from build123d import *

# Parameters (mm, degrees)
SKETCH1_W           = 15
SKETCH1_H           = 20
BOSS_EXTRUDE1_DEPTH = 20
FILLET1_R           = 7.5
CUT_EXTRUDE1_START  = -4.75
SKETCH3_R           = 8.5
CUT_EXTRUDE1_DEPTH  = 10.5
SKETCH4_R           = 2.5
CUT_EXTRUDE2_DEPTH  = 30.261749777
CUT_EXTRUDE3_DEPTH  = 3
SKETCH6_R           = 4
CUT_EXTRUDE4_DEPTH  = 3
CUT_EXTRUDE5_DEPTH  = 30.261749777
SKETCH8_R           = 8.5
CUT_EXTRUDE6_DEPTH  = 5
SKETCH9_R           = 2.5
CUT_EXTRUDE7_DEPTH  = 27.100766272
CUT_EXTRUDE8_START  = -1
CUT_EXTRUDE8_DEPTH  = 2.5
SKETCH11_R          = 1.5
CUT_EXTRUDE9_DEPTH  = 10
SKETCH12_W          = 15
SKETCH12_H          = 7
CUT_EXTRUDE10_DEPTH = 5
SKETCH13_W          = 15
SKETCH13_H          = 7
CUT_EXTRUDE11_DEPTH = 5
FILLET2_R           = 5


# Some blends are built 0.0001 mm under size
with BuildPart() as part:
    # Sketch1 → Boss-Extrude1 (new, symmetric)
    with BuildSketch(Plane.XY):
        Rectangle(SKETCH1_W, SKETCH1_H)
    extrude(amount=BOSS_EXTRUDE1_DEPTH, both=True)

    # Fillet1
    fillet1_edges = [part.edges().sort_by_distance(p)[0] for p in [
        (-7.5, 0, -20),
        (7.5, 0, -20),
    ]]
    fillet(fillet1_edges, radius=FILLET1_R - 0.0001)  # a hair under: the kernel refuses the full size

    # Sketch3 → Cut-Extrude1 (cut)
    with BuildSketch(Plane(origin=(0, 10, 0), x_dir=(1, 0, 0), z_dir=(0, 1, 0)).offset(CUT_EXTRUDE1_START)):
        with Locations((0, 12.5)):
            Circle(SKETCH3_R)
    extrude(amount=-CUT_EXTRUDE1_DEPTH, mode=Mode.SUBTRACT)

    # Sketch4 → Cut-Extrude2 (cut, through all)
    with BuildSketch(Plane(origin=(0, 10, 0), x_dir=(1, 0, 0), z_dir=(0, 1, 0))):
        with Locations(Location((0, 12.5, 0), (0, 0, 270))):
            Circle(SKETCH4_R)
    extrude(amount=-CUT_EXTRUDE2_DEPTH, mode=Mode.SUBTRACT)

    # Sketch5 → Cut-Extrude3 (cut)
    with BuildSketch(Plane(origin=(0, -10, 0), x_dir=(-1, 0, 0), z_dir=(0, -1, 0))):
        Polygon((-2.020725942, 16), (-4.041451884, 12.5), (-2.020725942, 9), (2.020725942, 9), (4.041451884, 12.5), (2.020725942, 16), align=None)
    extrude(amount=-CUT_EXTRUDE3_DEPTH, mode=Mode.SUBTRACT)

    # Sketch6 → Cut-Extrude4 (cut)
    with BuildSketch(Plane(origin=(0, 10, 0), x_dir=(1, 0, 0), z_dir=(0, 1, 0))):
        with Locations(Location((0, 12.5, 0), (0, 0, 270))):
            Circle(SKETCH6_R)
    extrude(amount=-CUT_EXTRUDE4_DEPTH, mode=Mode.SUBTRACT)

    # Sketch7 → Cut-Extrude5 (cut, through all)
    with BuildSketch(Plane.XZ.offset(10)):
        with BuildLine():
            Line((-7.5, 12.5), (-7.5, 22.5))
            Line((-7.5, 22.5), (7.5, 22.5))
            Line((7.5, 22.5), (7.5, 12.5))
            ThreePointArc((7.5, 12.5), (0, 20), (-7.5, 12.5))
        make_face()
    extrude(amount=-CUT_EXTRUDE5_DEPTH, mode=Mode.SUBTRACT)

    # Sketch8 → Cut-Extrude6 (cut)
    with BuildSketch(Plane.XZ.offset(10)):
        with Locations((0, 12.5)):
            Circle(SKETCH8_R)
    cut_extrude6 = extrude(amount=-CUT_EXTRUDE6_DEPTH, mode=Mode.SUBTRACT)

    # Mirror3: Cut-Extrude6 across plane
    add(cut_extrude6.mirror(Plane.ZX), mode=Mode.SUBTRACT)

    # Sketch9 → Cut-Extrude7 (cut, through all)
    with BuildSketch(Plane.XZ.offset(5)):
        with Locations(Location((0, 12.5, 0), (0, 0, 270))):
            Circle(SKETCH9_R)
    extrude(amount=-CUT_EXTRUDE7_DEPTH, mode=Mode.SUBTRACT)

    # Sketch10 → Cut-Extrude8 (cut)
    with BuildSketch(Plane(origin=(0, 10, 0), x_dir=(1, 0, 0), z_dir=(0, 1, 0)).offset(CUT_EXTRUDE8_START)):
        Polygon((1.58771324, 2.75), (7.5, 2.75), (7.5, 8.25), (1.58771324, 8.25), (-1.58771324, 8.25), (-3.175426481, 5.5), (-1.58771324, 2.75), align=None)
    extrude(amount=-CUT_EXTRUDE8_DEPTH, mode=Mode.SUBTRACT)

    # Sketch11 → Cut-Extrude9 (cut)
    with BuildSketch(Plane(origin=(0, 10, 0), x_dir=(1, 0, 0), z_dir=(0, 1, 0))):
        with Locations(Location((0, 5.5, 0), (0, 0, 270))):
            Circle(SKETCH11_R)
    extrude(amount=-CUT_EXTRUDE9_DEPTH, mode=Mode.SUBTRACT)

    # Sketch12 → Cut-Extrude10 (cut)
    with BuildSketch(Plane(origin=(0, 10, 0), x_dir=(1, 0, 0), z_dir=(0, 1, 0))):
        with Locations((0, -5)):
            Rectangle(SKETCH12_W, SKETCH12_H)
    extrude(amount=-CUT_EXTRUDE10_DEPTH, mode=Mode.SUBTRACT)

    # Sketch13 → Cut-Extrude11 (cut)
    with BuildSketch(Plane.XZ.offset(10)):
        with Locations((0, 5)):
            Rectangle(SKETCH13_W, SKETCH13_H)
    extrude(amount=-CUT_EXTRUDE11_DEPTH, mode=Mode.SUBTRACT)

    # Fillet2
    # the kernel refuses this fillet: 5 mm, written as the material it takes off along each edge
    with BuildSketch(Plane(origin=(-7.5, 22.5, 1.5), x_dir=(1, 0, 0), z_dir=(0, -1, 0)), Plane(origin=(7.5, -22.5, 1.5), x_dir=(-1, 0, 0), z_dir=(0, 1, 0)), Plane(origin=(-7.5, -22.5, 1.5), x_dir=(0, 0, -1), z_dir=(0, 1, 0))) as fillet2_piece_1:
        with BuildLine():
            CenterArc((FILLET2_R, -FILLET2_R), FILLET2_R, 90, 90)
            Line((0, -FILLET2_R), (0, 0))
            Line((0, 0), (FILLET2_R, 0))
        make_face()
    extrude(amount=17.5, mode=Mode.SUBTRACT)
    with BuildSketch(Plane(origin=(-7.5, 22.5, 1.5), x_dir=(1, 0, 0), z_dir=(0, -1, 0))) as fillet2_piece_2_section:
        with BuildLine():
            CenterArc((FILLET2_R, -FILLET2_R), FILLET2_R, 90, 90)
            Line((0, -FILLET2_R), (0, 0))
            Line((0, 0), (FILLET2_R, 0))
        make_face()
    fillet2_piece_2 = extrude(amount=30, mode=Mode.PRIVATE)
    fillet2_piece_2 = split(fillet2_piece_2, bisect_by=Plane(origin=(-6.368024429, -5, 0.368024429), z_dir=(0, -1, 0)), keep=Keep.TOP, mode=Mode.PRIVATE)
    add(fillet2_piece_2, mode=Mode.SUBTRACT)
    with BuildSketch(Plane(origin=(7.5, 22.5, 1.5), x_dir=(-1, 0, 0), z_dir=(0, -1, 0))) as fillet2_piece_3:
        with BuildLine():
            CenterArc((FILLET2_R, FILLET2_R), FILLET2_R, 180, 90)
            Line((0, FILLET2_R), (0, 0))
            Line((0, 0), (FILLET2_R, 0))
        make_face()
    extrude(amount=17.5, mode=Mode.SUBTRACT)
    with BuildSketch(Plane(origin=(7.5, 22.5, 1.5), x_dir=(-1, 0, 0), z_dir=(0, -1, 0))) as fillet2_piece_4_section:
        with BuildLine():
            CenterArc((FILLET2_R, FILLET2_R), FILLET2_R, 180, 90)
            Line((0, FILLET2_R), (0, 0))
            Line((0, 0), (FILLET2_R, 0))
        make_face()
    fillet2_piece_4 = extrude(amount=30, mode=Mode.PRIVATE)
    fillet2_piece_4 = split(fillet2_piece_4, bisect_by=Plane(origin=(6.368024429, -5, 0.368024429), z_dir=(0, -1, 0)), keep=Keep.TOP, mode=Mode.PRIVATE)
    add(fillet2_piece_4, mode=Mode.SUBTRACT)
    with BuildSketch(Plane(origin=(7.5, -22.5, 1.5), x_dir=(-1, 0, 0), z_dir=(0, 1, 0))) as fillet2_piece_5_section:
        with BuildLine():
            CenterArc((FILLET2_R, -FILLET2_R), FILLET2_R, 90, 90)
            Line((0, -FILLET2_R), (0, 0))
            Line((0, 0), (FILLET2_R, 0))
        make_face()
    fillet2_piece_5 = extrude(amount=30, mode=Mode.PRIVATE)
    fillet2_piece_5 = split(fillet2_piece_5, bisect_by=Plane(origin=(6.368024429, 5, 0.368024429), z_dir=(0, 1, 0)), keep=Keep.TOP, mode=Mode.PRIVATE)
    add(fillet2_piece_5, mode=Mode.SUBTRACT)
    with BuildSketch(Plane(origin=(-7.5, -22.5, 1.5), x_dir=(0, 0, -1), z_dir=(0, 1, 0))) as fillet2_piece_6_section:
        with BuildLine():
            CenterArc((FILLET2_R, -FILLET2_R), FILLET2_R, 90, 90)
            Line((0, -FILLET2_R), (0, 0))
            Line((0, 0), (FILLET2_R, 0))
        make_face()
    fillet2_piece_6 = extrude(amount=30, mode=Mode.PRIVATE)
    fillet2_piece_6 = split(fillet2_piece_6, bisect_by=Plane(origin=(-6.368024429, 5, 0.368024429), z_dir=(0, 1, 0)), keep=Keep.TOP, mode=Mode.PRIVATE)
    add(fillet2_piece_6, mode=Mode.SUBTRACT)


solid = part.part
For this review, take the finished solid that the model builds, in its own axes (mm). A direction names the side the tool comes from. Round coordinates to 2 decimals unless told otherwise and drop trailing zeros. Loops run counter-clockwise (first coordinate to the right, second up) from the corner with the lowest first, then second, coordinate; pieces in that order, holes last. Notation, with made-up numbers: (59.5, 14) - (64.5, 14) arc R33 ccw to (64.5, 52) - close; hole circle Ø2 at (-36, -33.75). An arc over 180 degrees is marked (long way). Put each result on its own line as item: value. Start each with the question number.
1. Consider section B-B on x = 6.25. State the section outline as (y, z) points, plus the area to 3 significant figures.
2. Consider section D-D on x = -0.75. State how many separate pieces and enclosed holes the cut face has, plus the area to 3 significant figures.
3. For faces 4 (the cylindrical face through (-6, 7.54, 0.07)), 5 (the flat face through (0, 8, 1.5)), 6 (the flat face through (3, 8, -8.25)), 7 (the cylindrical face through (-2.4, 8.5, -15.7)), 8 (the flat face through (0, -9, -16)), list the 3-axis set-ups (+Z, -Z, +X, -X, +Y, -Y) from which the entire face can be reached by the end or side of a thin tool; tool diameter is ignored.
4. Mouldability with a two-part tool opening along X and no side actions: class faces 1 (the cylindrical face through (0, 0, 15)), 2 (the cylindrical face through (6, -7.54, 0.07)), 3 (the flat face through (3, 8, -2.75)) as +X half, -X half, draft (parallel to the pull), parting line (faces both ways), or undercut.
5. Insertion check: P1, Ø3, axis at x = 0, z = 12.5, coming from the +Y side; P2, Ø2, axis at x = -1.5, y = 3, coming from the -Z side; P3, Ø2.5, axis at x = 1, y = -7, coming from the +Z side; P4, Ø3, axis at x = -4.5, z = 9, coming from the +Y side. Each pin has a flat end and moves straight along its axis. Give the tip position at first contact, or say it passes through.
6. For probe 1 along Y at (x, z) = (2.5, -3.5); probe 2 along Y at (x, z) = (1.5, -5); probe 3 along Y at (x, z) = (-3.25, -10), list the stretches that pass through material, from the lowest coordinate up. Write a range as [from, to].
7. Consider section C-C on y = 2. State the section outline as (x, z) points.
Result sheet:
1. outline: (-10, -16.65) - (-5.25, -16.65) - (-5.25, -6.74) - (5.25, -6.74) - (5.25, -16.65) - (10, -16.65) - (10, -0.19) - (5, -0.19) - (5, 16.65) - (-5, 16.65) - (-5, -0.19) - (-10, -0.19) - close; hole (6.5, -8.25) - (9, -8.25) - (9, -2.75) - (6.5, -2.75) - close
1. area: 380 mm^2
2. separate pieces: 5
2. enclosed holes: 0
2. area: 318 mm^2
3. face 4: +Z, -X, +Y
3. face 5: +Z, +X, -X, +Y
3. face 6: +X
3. face 7: +Y
3. face 8: -Y
4. face 1: undercut
4. face 2: +X half
4. face 3: draft
5. P1: through
5. P2: z = -4.38
5. P3: z = 1.5
5. P4: y = 5
6. probe 1: [-10, 6.5], [9, 10]
6. probe 2: [-10, -5.25], [5.25, 6.5], [9, 10]
6. probe 3: [-10, -5.25], [5.25, 10]
7. outline: (-7.5, -8.5) arc R8.5 cw to (7.5, -8.5) - (7.5, 12.5) arc R7.5 ccw to (-7.5, 12.5) - close; hole circle Ø5 at (0, 12.5)
